```python
from build123d import *

# Parameters (mm, degrees)
SKETCH1_W                                = 66
SKETCH1_H                                = 80
BOSS_EXTRUDE1_DEPTH                      = 6
CBORE_FOR_M2_5_SHCS2_D                   = 2.9
CBORE_FOR_M2_5_SHCS2_CBORE_D             = 5.5
CBORE_FOR_M2_5_SHCS2_CBORE_DEPTH         = 2.5
BOSS_EXTRUDE2_DEPTH                      = 80
RIB1_REACH                               = 101.785
SKETCH5_WALL_W                           = 278.74466228
SKETCH5_WALL_H                           = 6
CBORE_FOR_M4_SHCS1_D                     = 4.5
CBORE_FOR_M4_SHCS1_CBORE_D               = 8
CBORE_FOR_M4_SHCS1_CBORE_DEPTH           = 4
CBORE_FOR_M4_SHCS1_ON_FACE_2_D           = 4.5
CBORE_FOR_M4_SHCS1_ON_FACE_2_CBORE_D     = 8
CBORE_FOR_M4_SHCS1_ON_FACE_2_CBORE_DEPTH = 4


with BuildPart() as part:
    # Sketch1 → Boss-Extrude1 (new body)
    with BuildSketch(Plane(origin=(0, 0, 0), x_dir=(1, 0, 0), z_dir=(0, 1, 0))):
        Rectangle(SKETCH1_W, SKETCH1_H)
    extrude(amount=BOSS_EXTRUDE1_DEPTH)

    # CBORE for M2.5 SHCS2 (through all)
    with Locations(Plane(origin=(0, 6, 0), x_dir=(1, 0, 0), z_dir=(0, 1, 0))):
        with Locations((20, -35), (-28, 35), (28, 35), (-20, -35)):
            CounterBoreHole(CBORE_FOR_M2_5_SHCS2_D / 2, CBORE_FOR_M2_5_SHCS2_CBORE_D / 2, CBORE_FOR_M2_5_SHCS2_CBORE_DEPTH)

    # Sketch4 → Boss-Extrude2 (add)
    with BuildSketch(Plane.XY.offset(40)):
        Polygon((-33, 0), (-33, 46), (-39, 46), (-39, 6), (-79, 6), (-79, 0), align=None)
    extrude(amount=-BOSS_EXTRUDE2_DEPTH)

    # Sketch5 wall → Rib1 (add, up to next)
    with BuildSketch(Plane(origin=(0, 26, 0), x_dir=(0.855197831554, -0.518301716093, 0), z_dir=(0.518301716093, 0.855197831554, 0)), mode=Mode.PRIVATE) as rib1_sk1:
        Rectangle(SKETCH5_WALL_W, SKETCH5_WALL_H)
    rib1_tool1 = extrude(rib1_sk1.sketch, amount=-RIB1_REACH, mode=Mode.PRIVATE) - part.part
    add(rib1_tool1.solids().sort_by_distance((0, 26, 0))[0])

    # CBORE for M4 SHCS1 (through all)
    with Locations(Plane(origin=(-59, 0, -20), x_dir=(0, 0, -1), z_dir=(0, -1, 0))):
        with Locations((0, 0), (-40, 0)):
            CounterBoreHole(CBORE_FOR_M4_SHCS1_D / 2, CBORE_FOR_M4_SHCS1_CBORE_D / 2, CBORE_FOR_M4_SHCS1_CBORE_DEPTH)

    # CBORE for M4 SHCS1 on face 2 (through all)
    with Locations(Plane(origin=(-33, 26, -21.5), x_dir=(0, 0, 1), z_dir=(1, 0, 0))):
        with Locations((0, 0), (43, 0)):
            CounterBoreHole(CBORE_FOR_M4_SHCS1_ON_FACE_2_D / 2, CBORE_FOR_M4_SHCS1_ON_FACE_2_CBORE_D / 2, CBORE_FOR_M4_SHCS1_ON_FACE_2_CBORE_DEPTH)


solid = part.part
```
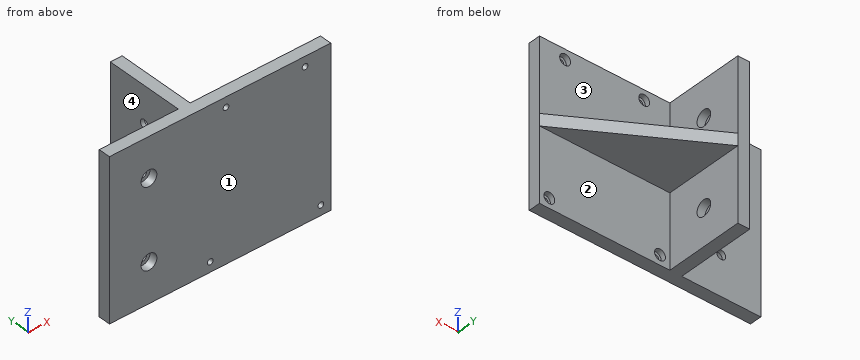
Here's how the part is built. I have some questions about the finished solid (model axes, mm). Face numbers are marked on the shaded views. A direction names the side the tool comes from. Coordinates: 2 decimals unless noted, no trailing zeros. Loops run counter-clockwise (first coordinate to the right, second up) from the corner with the lowest first, then second, coordinate; pieces in that order, holes last. Notation, with made-up numbers: M 60,62.25 L 70,62.25 A34 ccw 70,97.25 Z; hole C 41.25,-39.75 d9. An arc over 180 degrees is marked long. One line per item, written item: value.
1. Imagine slicing it at C-C (x = -20). List the corners of the cut face in (y, z) for me.
Geometry says:
outline: M 0,-40 L 6,-40 L 6,-3 L 38.12,-3 L 38.12,3 L 6,3 L 6,32.25 L 3.5,32.25 L 3.5,33.55 L 0,33.55 Z; M 0,36.45 L 3.5,36.45 L 3.5,37.75 L 6,37.75 L 6,40 L 0,40 Z
2. Please list where these lines run through material, in increasing order: probe 1 along Z at (x, y) = (-36, 26); probe 2 along Z at (x, y) = (-37.45, 26); probe 3 along X at (y, z) = (4.3, 35).
Geometry says:
probe 1: z = -40 to -25.5, -17.5 to 17.5, 25.5 to 40
probe 2: z = -40 to -23.75, -19.25 to 19.25, 23.75 to 40
probe 3: x = -79 to -22.75, -17.25 to 17.25, 22.75 to 33
3. Will these pins go through, and if not, where does the flat tip stop? pin 1 Ø10 at (y, z) = (36, 25.5) entering from +X; pin 2 Ø12 at (x, y) = (6, 25.5) entering from -Z; pin 3 Ø6.5 at (y, z) = (26, 22) entering from +X.
Geometry says:
pin 1: stops at x = -33
pin 2: stops at z = -3
pin 3: stops at x = -37
4. Imagine slicing it at D-D (y = 38). List the corners of the cut face in (x, z) for me, and give its area (3 significant figures).
Geometry says:
outline: M -39,-40 L -33,-40 L -33,-3 L -19.8,-3 L -19.8,3 L -33,3 L -33,40 L -39,40 Z
area: 559 mm2
5. On a 3-axis mill with a long thin cutter (end or side, diameter ignored), from which of +Z, -Z, +X, -X, +Y, -Y can I reach the whole of each face in a straight line? I mean the marked faces 1, 2, 3 and 4. Say none if no direction works.
Geometry says:
face 1: +Z, -Z, +X, -X, -Y
face 2: -Z, +X, +Y
face 3: +Z, +X, +Y
face 4: +Z, -Z, -X, +Y
6. Imagine slicing it at B-B (z = 35). List the corners of the cut face in (x, y) for me.
Geometry says:
outline: M -79,0 L -21.45,0 L -21.45,3.5 L -22.75,3.5 L -22.75,6 L -33,6 L -33,46 L -39,46 L -39,6 L -79,6 Z; M -18.55,0 L 18.55,0 L 18.55,3.5 L 17.25,3.5 L 17.25,6 L -17.25,6 L -17.25,3.5 L -18.55,3.5 Z; M 21.45,0 L 33,0 L 33,6 L 22.75,6 L 22.75,3.5 L 21.45,3.5 Z
7. Imagine slicing it at A-A (y = 26). List the corners of the cut face in (x, z) for me.
Geometry says:
outline: M -39,-40 L -33,-40 L -33,-25.5 L -37,-25.5 L -37,-23.75 L -39,-23.75 Z; M -39,-19.25 L -37,-19.25 L -37,-17.5 L -33,-17.5 L -33,-3 L 0,-3 L 0,3 L -33,3 L -33,17.5 L -37,17.5 L -37,19.25 L -39,19.25 Z; M -39,23.75 L -37,23.75 L -37,25.5 L -33,25.5 L -33,40 L -39,40 Z
